Source: CAD feature listing. Evaluate the final solid. Frame: model axes, mm. Face numbers are marked on the shaded views. A direction names the side the tool comes from. Give positions to 0.01 mm unless a question says otherwise; leave off trailing zeros. Loops run counter-clockwise (first coordinate to the right, second up) from the corner with the lowest first, then second, coordinate; pieces in that order, holes last.
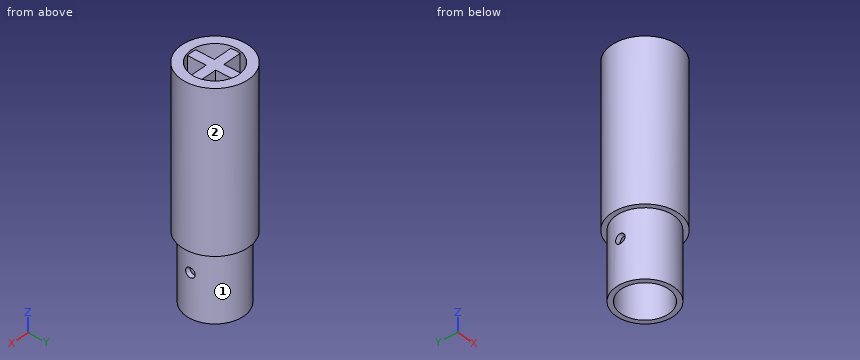
```python
from build123d import *

# Parameters (mm, degrees)
F1_R      = 14
F1_R_2    = 10
F2_DEPTH  = 60
F4_DEPTH  = 59
F6_R      = 14
F7_DEPTH  = 6
F8_R      = 3.5
F8_R_2    = 2.25
F9_DEPTH  = 1.5
F10_R     = 12
F10_R_2   = 10
F11_DEPTH = 28
F12_R     = 2
F13_DEPTH = 12.5
F14_DEPTH = 34.0010001


with BuildPart() as f2:
    # F1 (on face) → F2 (new body)
    with BuildSketch(Plane.XY):
        Circle(F1_R)
        Circle(F1_R_2, mode=Mode.SUBTRACT)
    extrude(amount=F2_DEPTH)

    # F3 (on Top) → F4 (join)
    with BuildSketch(Plane.XY):
        with BuildLine():
            ThreePointArc((2, 9.7979589711), (0, 10), (-2, 9.7979589711))
            Line((-2, 9.7979589711), (-2, 2))
            Line((-2, 2), (-9.7979589711, 2))
            ThreePointArc((-9.7979589711, 2), (-10, 0), (-9.7979589711, -2))
            Line((-9.7979589711, -2), (-2, -2))
            Line((-2, -2), (-2, -9.7979589711))
            ThreePointArc((-2, -9.7979589711), (-1.0050896201, -9.9493615301), (0, -10))
            ThreePointArc((0, -10), (1.0050896201, -9.9493615301), (2, -9.7979589711))
            Line((2, -9.7979589711), (2, -2))
            Line((2, -2), (9.7979589711, -2))
            ThreePointArc((9.7979589711, -2), (10, 0), (9.7979589711, 2))
            Line((9.7979589711, 2), (2, 2))
            Line((2, 2), (2, 9.7979589711))
        make_face()
    extrude(amount=F4_DEPTH)

    # F6 (on Top) → F7 (join)
    with BuildSketch(Plane.XY):
        Circle(F6_R)
        with BuildLine():
            ThreePointArc((-9.7979589711, 2), (-7.0710678119, 7.0710678119), (-2, 9.7979589711))
            Line((-2, 9.7979589711), (-2, 2))
            Line((-2, 2), (-9.7979589711, 2))
        make_face(mode=Mode.SUBTRACT)
    extrude(amount=-F7_DEPTH)

    # F8 (on face) → F9 (cut)
    with BuildSketch(Plane(origin=(0, 0, -6), x_dir=(1, 0, 0), z_dir=(0, 0, -1))):
        Circle(F8_R)
        Circle(F8_R_2, mode=Mode.SUBTRACT)
    extrude(amount=-F9_DEPTH, mode=Mode.SUBTRACT)

    # F10 (on face) → F11 (join)
    with BuildSketch(Plane(origin=(0, 0, -6), x_dir=(1, 0, 0), z_dir=(0, 0, -1))):
        Circle(F10_R)
        Circle(F10_R_2, mode=Mode.SUBTRACT)
    extrude(amount=F11_DEPTH)

    # F12 (on Right) → F13 (cut, symmetric)
    with BuildSketch(Plane.YZ):
        with Locations((0, -16)):
            Circle(F12_R)
    extrude(amount=F13_DEPTH, both=True, mode=Mode.SUBTRACT)

    # F6 (on Top) → F14 (cut, through all)
    with BuildSketch(Plane.XY):
        with BuildLine():
            Line((-2, 2), (-2, 9.7979589711))
            ThreePointArc((-2, 9.7979589711), (-7.0710678119, 7.0710678119), (-9.7979589711, 2))
            Line((-9.7979589711, 2), (-2, 2))
        make_face()
    extrude(amount=-F14_DEPTH, mode=Mode.SUBTRACT)


solid = f2.part
```
(1) Section A-A, the plane y = 0. Count the separate pieces of the cut face and the enclosed holes in it, then the cut area to 3 significant figures.
A:
separate pieces: 3
enclosed holes: 0
area: 1,920 mm2
(2) Section B-B, the plane x = 0. Return the cut outline in (y, z).
A:
outline: (-14, -6) - (-12, -6) - (-12, -34) - (-10, -34) - (-10, -6) - (-3.5, -6) - (-3.5, -4.5) - (-2.25, -4.5) - (-2.25, -6) - (2.25, -6) - (2.25, -4.5) - (3.5, -4.5) - (3.5, -6) - (10, -6) - (10, -34) - (12, -34) - (12, -6) - (14, -6) - (14, 60) - (10, 60) - (10, 59) - (-10, 59) - (-10, 60) - (-14, 60) - close
(3) Ray query, line 1 along Y through (x, z) = (0, -4.9); line 2 along X through (y, z) = (-9, 11.5); line 3 along Y through (x, z) = (8.25, 11.5). Return the intervals inside material, ascending.
A:
line 1: y = -14 to -3.5, -2.25 to 2.25, 3.5 to 14
line 2: x = -10.72 to -4.36, -2 to 2, 4.36 to 10.72
line 3: y = -11.31 to -5.65, -2 to 2, 5.65 to 11.31
(4) Reachability of the marked faces 1 and 2 from +Z, -Z, +X, -X, +Y, -Y: full face, straight path, thin tool, end or side. Return the list, or none.
A:
face 1: -Z
face 2: +Z, -Z
(5) First-contact query: pin 1 (6 mm diameter, centred on x = -5.5, z = 35, fed in from -Y) (3 decimals); pin 2 (5 mm diameter, centred on y = 0, z = -16, fed in from -X); pin 3 (2 mm diameter, centred on y = 9.5, z = -9.5, fed in from +X). Flat tips, straight axial feed; report the tip coordinate or a pass-through.
A:
pin 1: stops at y = -13.775
pin 2: stops at x = -12
pin 3: stops at x = 8.47
(6) Section D-D, the plane y = 5. Return the cut outline in (x, z), then the cut area to 3 significant figures.
A:
outline: (-13.08, -6) - (-10.91, -6) - (-10.91, -34) - (-8.66, -34) - (-8.66, 60) - (-13.08, 60) - close; (-2, -6) - (8.66, -6) - (8.66, -34) - (10.91, -34) - (10.91, -6) - (13.08, -6) - (13.08, 60) - (8.66, 60) - (8.66, 0) - (2, 0) - (2, 59) - (-2, 59) - close
area: 1,010 mm2
(7) Section C-C, the plane z = 10.5. Return the cut outline in (x, y).
A:
outline: circle Ø28 at (0, 0); hole (-9.8, -2) arc R10 ccw to (-2, -9.8) - (-2, -2) - close; hole (-9.8, 2) - (-2, 2) - (-2, 9.8) arc R10 ccw to start; hole (2, -9.8) arc R10 ccw to (9.8, -2) - (2, -2) - close; hole (2, 2) - (9.8, 2) arc R10 ccw to (2, 9.8) - close
